Geometry check sheet. Reference: the model listing, model coordinates, mm. Face numbers are marked on the shaded views. Coordinates: 2 decimals unless noted, no trailing zeros. Order: outer loops, then holes, each group sorted by start corner. A loop starts at its lowest first (then second) coordinate and runs counter-clockwise, first axis right, second up. Notation, with made-up numbers: M 33.25,7.5 L 63.25,7.5 A12 ccw 63.25,30.5 Z; hole C 58.5,49 d11. An arc over 180 degrees is marked long. One line per item, written item: value. Start each with the question number.
1) Draft check along X on the marked faces 1 and 2. Enter one of: pulls with the +X half, pulls with the -X half, needs draft (parallel to the pull), parting line crosses it, or undercut.
2) Sectioned sample at C-C, the plane y = -69. Enter the section's corners in (x, z), then the cut area to 3 significant figures.
3) Sectioned sample at A-A, the plane z = 0. Enter the section's corners in (x, y).
4) Go/stop test with flat-tipped pins: P1, Ø1.5, axis at x = 0, z = 1, coming from the -Y side; P2, Ø6, axis at x = 4, y = -86, coming from the +Z side; P3, Ø8, axis at y = -74, z = -3.5, coming from the +X side. Record where each tip stops, or that it passes through.
5) Thickness scan on L1, parallel to X at y = -30.5, z = 0.5; L2, parallel to Y at x = -1.5, z = -1.75; L3, parallel to Z at x = 0.25, y = -98.5. Record the ranges inside material, lowest first. Write a range as from..to.
6) Sectioned sample at B-B, the plane x = 0. Enter the section's corners in (y, z).
```python
from build123d import *

# Parameters (mm, degrees)
SKETCH1_R           = 2.5
BOSS_EXTRUDE1_DEPTH = 20
SKETCH2_R           = 4.5
BOSS_EXTRUDE2_DEPTH = 30
FILLET1_R           = 2


with BuildPart() as part:
    # Sketch1 → Boss-Extrude1 (new body)
    with BuildSketch(Plane(origin=(0, 0, 0), x_dir=(1, 0, 0), z_dir=(0, 1, 0))):
        with Locations(Location((0, 0, 0), (0, 0, 270))):
            Circle(SKETCH1_R)
    extrude(amount=BOSS_EXTRUDE1_DEPTH)

    # Sketch2 → Boss-Extrude2 (add)
    with BuildSketch(Plane.XZ):
        with Locations(Location((0, 0, 0), (0, 0, 270))):
            Circle(SKETCH2_R)
    extrude(amount=BOSS_EXTRUDE2_DEPTH)

    # Sketch3 → Revolve1 (revolve)
    with BuildSketch(Plane.XY, mode=Mode.PRIVATE) as revolve1_sk:
        Polygon((10, -105), (4.5, -30), (2.5, -30), (7.25, -105), align=None)
    revolve(revolve1_sk.sketch.rotate(Axis((0, -30, 0), (0, -1, 0)), 270), axis=Axis((0, -30, 0), (0, -1, 0)))

    # Fillet1
    fillet1_edges = [part.edges().sort_by_distance(p)[0] for p in [
        (0, -105, 10),
    ]]
    fillet(fillet1_edges, radius=FILLET1_R)


solid = part.part
```
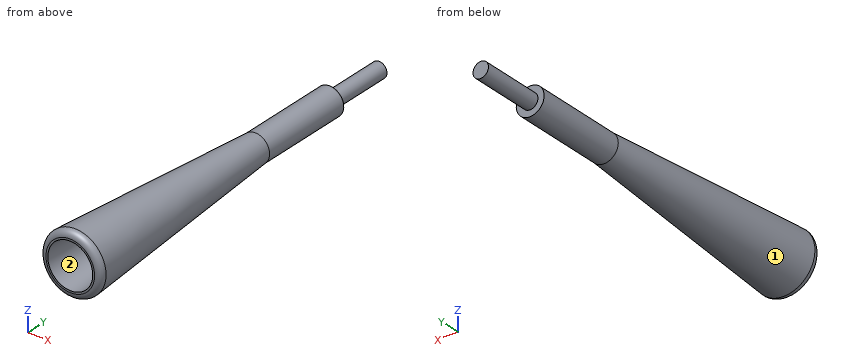
Final values:
1. face 1: parting line crosses it
1. face 2: undercut
2. outline: C 0,0 d14.72; hole C 0,0 d9.94
2. area: 92.6 mm^2
3. outline: M -9.84,-102.85 A2 ccw -7.85,-105 L -7.25,-105 L -2.5,-30 L 2.5,-30 L 7.25,-105 L 7.85,-105 A2 ccw 9.84,-102.85 L 4.5,-30 L 4.5,0 L 2.5,0 L 2.5,20 L -2.5,20 L -2.5,0 L -4.5,0 L -4.5,-30 Z
4. P1: stops at y = -30
4. P2: stops at z = 8.6
4. P3: stops at x = 7.91
5. L1: x = -4.51..-2.48, 2.48..4.51
5. L2: y = -30..20
5. L3: z = -9.52..-6.83, 6.83..9.52
6. outline: M -105,-7.85 A2 ccw -102.85,-9.84 L -30,-4.5 L 0,-4.5 L 0,-2.5 L 20,-2.5 L 20,2.5 L 0,2.5 L 0,4.5 L -30,4.5 L -102.85,9.84 A2 ccw -105,7.85 L -105,7.25 L -30,2.5 L -30,-2.5 L -105,-7.25 Z
